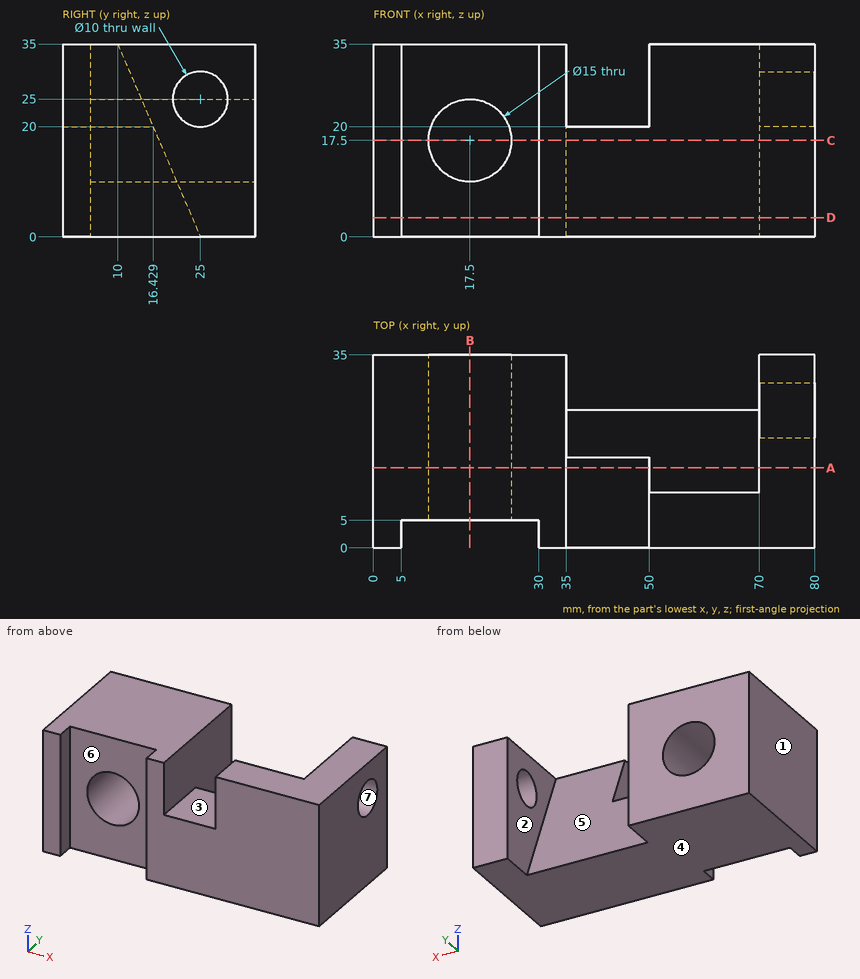
Source: three-view drawing plus pictorial views. Frame: mm from the lowest corner of the part. A direction names the side the tool comes from. Coordinates: 2 decimals unless noted, no trailing zeros. Loops run counter-clockwise (first coordinate to the right, second up) from the corner with the lowest first, then second, coordinate; pieces in that order, holes last. Notation, with made-up numbers: M -3.5,87.5 L 34.5,87.5 A30 cw 34.5,115.5 Z; hole C -7.5,-24.5 d2. An arc over 180 degrees is marked long. Use CSV: the item, a comma, the result in double quotes.
(1) Line query: line 1 (X direction, y = 29.25, z = 17.5); line 2 (X direction, y = 2, z = 25); line 3 (Z direction, x = 17.5, y = 19). Output: solid intervals per line, ascending. Write a range as [from, to].
Answers follow:
line 1,"[0, 10], [25, 35], [70, 80]"
line 2,"[0, 5], [30, 35], [50, 80]"
line 3,"[0, 10], [25, 35]"
(2) Contact query for a flat-ended pin moving along its axis: pin 1 (9 mm diameter, centred on y = 25, z = 25, fed in from +X). Output: stop coordinate, or through.
Answers follow:
pin 1,"x = 35"
(3) Cut plane C-C on z = 17.5. Return loops of the section in (x, y), and give its area (3 significant figures).
Answers follow:
outline,"M 0,0 L 5,0 L 5,5 L 10,5 L 10,35 L 0,35 Z; M 25,5 L 30,5 L 30,0 L 80,0 L 80,35 L 70,35 L 70,17.5 L 35,17.5 L 35,35 L 25,35 Z"
area,"1,610 mm²"
(4) Cut plane A-A on y = 14.5. Return loops of the section in (x, z).
Answers follow:
outline,"M 0,0 L 80,0 L 80,35 L 70,35 L 70,24.5 L 50,24.5 L 50,20 L 35,20 L 35,35 L 0,35 Z; hole C 17.5,17.5 d15"
(5) Cut plane B-B on x = 17.5. Return loops of the section in (y, z), and give its area (3 significant figures).
Answers follow:
outline,"M 5,0 L 35,0 L 35,10 L 5,10 Z; M 5,25 L 35,25 L 35,35 L 5,35 Z"
area,"600 mm²"
(6) Cut plane D-D on z = 3.5. Return loops of the section in (x, y), and give its area (3 significant figures).
Answers follow:
outline,"M 0,0 L 5,0 L 5,5 L 30,5 L 30,0 L 80,0 L 80,35 L 70,35 L 70,23.5 L 35,23.5 L 35,35 L 0,35 Z"
area,"2,270 mm²"
(7) Reachability of the marked faces 1, 2 and 3 from +Z, -Z, +X, -X, +Y, -Y: full face, straight path, thin tool, end or side. Return the list, or none.
Answers follow:
face 1,"+Z, -Z, -X, +Y, -Y"
face 2,"+Z, +Y"
face 3,"+Z, +Y, -Y"
(8) Draft query along Z for the marked faces 4, 5, 6 and 7. Return one class per face: pulls with the +Z half, pulls with the -Z half, needs draft (parallel to the pull), parting line crosses it, or undercut.
Answers follow:
face 4,"pulls with the -Z half"
face 5,"pulls with the +Z half"
face 6,"needs draft"
face 7,"undercut"
